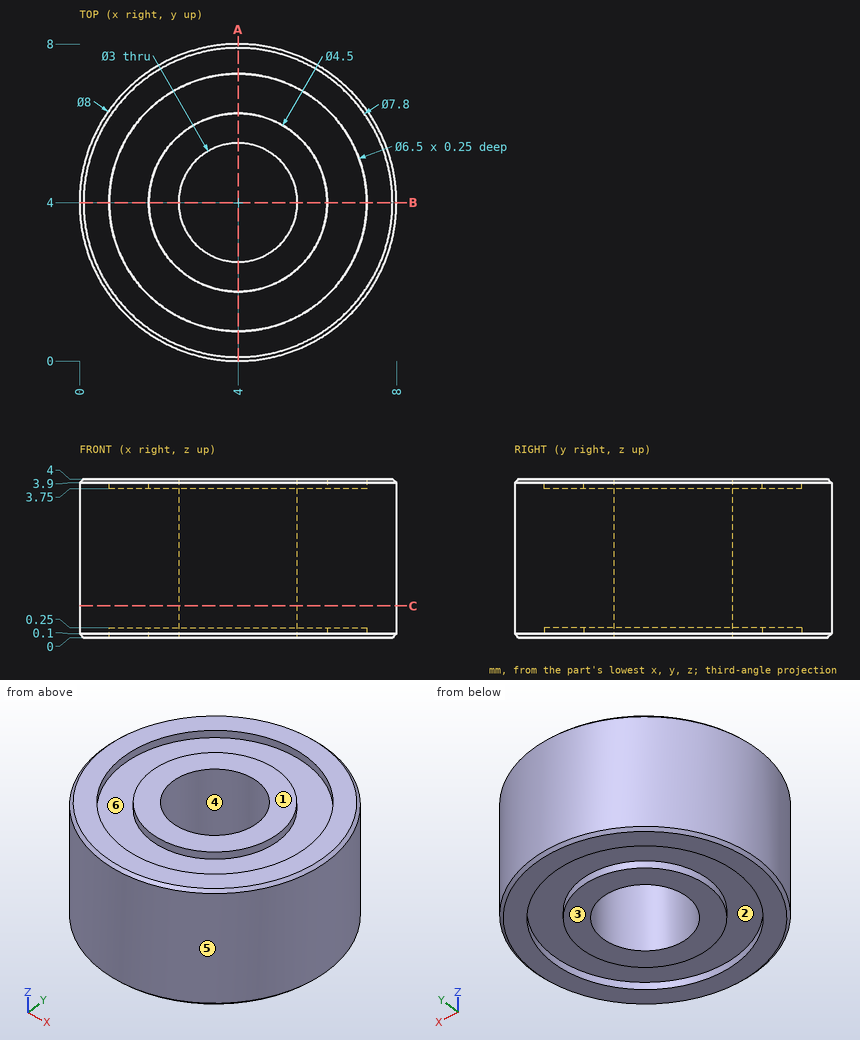
Source: three-view drawing plus pictorial views. Frame: mm from the lowest corner of the part. A direction names the side the tool comes from. Round coordinates to 2 decimals unless told otherwise and drop trailing zeros. Order: outer loops, then holes, each group sorted by start corner. A loop starts at its lowest first (then second) coordinate and runs counter-clockwise, first axis right, second up. Notation, with made-up numbers: (1.25, 8) -> (51.25, 8) arc R11 ccw to (51.25, 14) -> close; hole circle Ø10 at (76.5, -1.75). An arc over 180 degrees is marked (long way). Use one line per item in the form item = value. Start each with the question number.
1. Reachability of the marked faces 1 and 2 from +Z, -Z, +X, -X, +Y, -Y: full face, straight path, thin tool, end or side. Return the list, or none.
2. Pin query (flat end, axial travel): pin 1 Ø2 at (x, z) = (1.5, 3) entering from -Y. Return the tip coordinate at first contact, or that it passes through.
3. Draft query along X for the marked faces 3, 4, 5 and 6. Return one class per face: pulls with the +X half, pulls with the -X half, needs draft (parallel to the pull), parting line crosses it, or undercut.
4. Line query: probe 1 along Y at (x, z) = (4, 0.2); probe 2 along Y at (x, z) = (4, 3.95); probe 3 along X at (y, z) = (3, 2.1). Output: solid intervals per line, ascending.
5. Cut plane A-A (x = 4). Return the cut outline in (y, z), then the cut area to 3 significant figures.
6. Cut plane C-C (z = 0.8). Return the cut outline in (x, y).
Solution:
q1.face_1 = +Z, +X, -X, +Y, -Y
q1.face_2 = -Z
q2.pin_1 = 0.29
q3.face_3 = needs draft
q3.face_4 = undercut
q3.face_5 = parting line crosses it
q3.face_6 = undercut
q4.probe_1 = 0 to 0.75, 1.75 to 2.5, 5.5 to 6.25, 7.25 to 8
q4.probe_2 = 0.05 to 0.75, 1.75 to 2.5, 5.5 to 6.25, 7.25 to 7.95
q4.probe_3 = 0.13 to 2.88, 5.12 to 7.87
q5.outline = (0, 0.1) -> (0.1, 0) -> (0.75, 0) -> (0.75, 0.25) -> (1.75, 0.25) -> (1.75, 0) -> (2.5, 0) -> (2.5, 4) -> (1.75, 4) -> (1.75, 3.75) -> (0.75, 3.75) -> (0.75, 4) -> (0.1, 4) -> (0, 3.9) -> close; (5.5, 0) -> (6.25, 0) -> (6.25, 0.25) -> (7.25, 0.25) -> (7.25, 0) -> (7.9, 0) -> (8, 0.1) -> (8, 3.9) -> (7.9, 4) -> (7.25, 4) -> (7.25, 3.75) -> (6.25, 3.75) -> (6.25, 4) -> (5.5, 4) -> close
q5.area = 19.0 mm^2
q6.outline = circle Ø8 at (4, 4); hole circle Ø3 at (4, 4)
